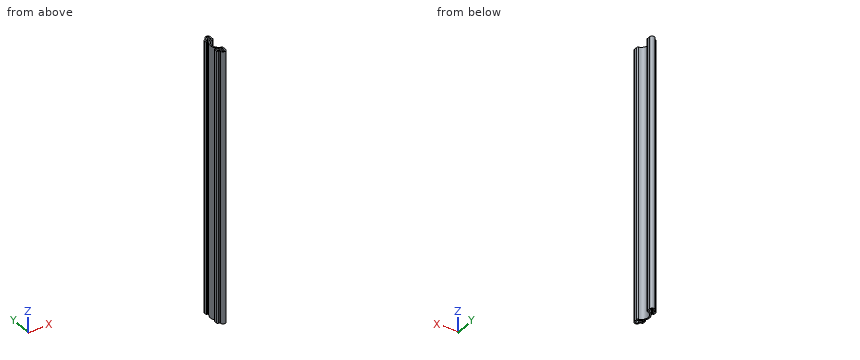
from build123d import *

# Parameters (mm, degrees)
EXTRUDE_THIN1_DEPTH = 254
FILLET1_R           = 1.27


with BuildPart() as part:
    # Sketch1 → Extrude-Thin1 (new body)
    with BuildSketch(Plane.XY):
        with BuildLine():
            Line((-7.14375, 7.14375), (-7.14375, 3.175))
            Line((-7.14375, 3.175), (-4.7625, 3.175))
            Line((-4.7625, 3.175), (-4.7625, 2.38125))
            ThreePointArc((-4.7625, 2.38125), (-2.38125, 0), (0, 2.38125))
            Line((0, 2.38125), (0, 6.35))
            ThreePointArc((0, 6.35), (-5.74675, 12.7), (0, 19.05))
            Line((0, 19.05), (0, 23.01875))
            ThreePointArc((0, 23.01875), (-2.38125, 25.4), (-4.7625, 23.01875))
            Line((-4.7625, 23.01875), (-4.7625, 22.225))
            Line((-4.7625, 22.225), (-7.14375, 22.225))
            Line((-7.14375, 22.225), (-7.14375, 18.25625))
            Line((-7.14375, 18.25625), (-5.87375, 18.25625))
            Line((-5.87375, 18.25625), (-5.87375, 20.955))
            Line((-5.87375, 20.955), (-3.4925, 20.955))
            Line((-3.4925, 20.955), (-3.4925, 23.01875))
            ThreePointArc((-3.4925, 23.01875), (-2.38125, 24.13), (-1.27, 23.01875))
            Line((-1.27, 23.01875), (-1.27, 20.110751986))
            ThreePointArc((-1.27, 20.110751986), (-7.01675, 12.7), (-1.27, 5.289248014))
            Line((-1.27, 5.289248014), (-1.27, 2.38125))
            ThreePointArc((-1.27, 2.38125), (-2.38125, 1.27), (-3.4925, 2.38125))
            Line((-3.4925, 2.38125), (-3.4925, 4.445))
            Line((-3.4925, 4.445), (-5.87375, 4.445))
            Line((-5.87375, 4.445), (-5.87375, 7.14375))
            Line((-5.87375, 7.14375), (-7.14375, 7.14375))
        make_face()
    extrude(amount=-EXTRUDE_THIN1_DEPTH)

    # Fillet1
    fillet1_edges = [part.edges().sort_by_distance(p)[0] for p in [
        (-3.4925, 4.445, -127),
        (-3.4925, 20.955, -127),
        (-7.14375, 22.225, -127),
        (0, 19.05, -127),
        (0, 6.35, -127),
        (-7.14375, 3.175, -127),
    ]]
    fillet(fillet1_edges, radius=FILLET1_R)


solid = part.part
Geometry check sheet. Reference: the model listing, model coordinates, mm. Round coordinates to 2 decimals unless told otherwise and drop trailing zeros. Loops run counter-clockwise (first coordinate to the right, second up) from the corner with the lowest first, then second, coordinate; pieces in that order, holes last.
Item 1: Cross-section at B-B on y = 10.75. Record the boundary of the cut face in (x, z), then the cut area to 3 significant figures.
Item 2: Thickness scan on line 1 (Y direction, x = -2, z = -69); line 2 (Y direction, x = -6, z = -193.5); line 3 (Y direction, x = -1.75, z = -116). Record the ranges inside material, lowest first.
Item 3: Gauge pin test, flat ends, axial feed: pin 1 (0.9 mm diameter, centred on y = 2.5, z = -184.5, fed in from -X); pin 2 (1.5 mm diameter, centred on x = -1.5, y = 22.5, fed in from +Z); pin 3 (3 mm diameter, centred on y = 13, z = -98, fed in from +X); pin 4 (1.5 mm diameter, centred on y = 3.5, z = -186, fed in from -X). Record the tip position at first contact, or that the pin passes through.
Answer sheet:
1. outline: (-6.76, -254) - (-5.44, -254) - (-5.44, 0) - (-6.76, 0) - close
1. area: 336 mm2
2. line 1: y = 0.03 to 1.34, 5.52 to 6.89, 18.51 to 19.88, 24.06 to 25.37
2. line 2: y = 3.18 to 7.14, 8.89 to 16.51, 18.26 to 22.22
2. line 3: y = 0.09 to 1.47, 5.43 to 6.78, 18.62 to 19.97, 23.93 to 25.31
3. pin 1: stops at x = -4.76
3. pin 2: stops at z = 0
3. pin 3: stops at x = -5.49
3. pin 4: stops at x = -7.13
